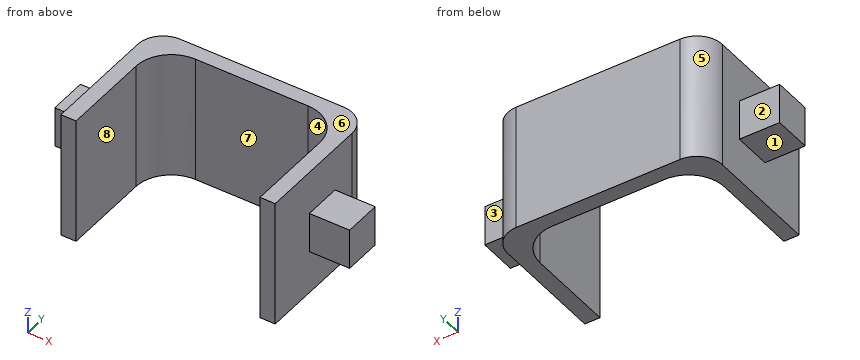
from build123d import *

# Parameters (mm, degrees)
BOSS_EXTRUDE1_DEPTH = 1.5875
BOSS_EXTRUDE2_DEPTH = 5
FILLET1_R           = 2
FILLET2_R           = 2
CUT_EXTRUDE1_DEPTH  = 10


with BuildPart() as part:
    # Sketch1 → Boss-Extrude1 (new body, symmetric)
    with BuildSketch(Plane.XY):
        Polygon((8.45, 11), (8.45, 7), (11.625, 7), (11.625, 4), (8.45, 4), (8.45, 0), (6.45, 0), (6.45, 9), (-6.45, 9), (-6.45, 0), (-8.45, 0), (-8.45, 4), (-11.625, 4), (-11.625, 7), (-8.45, 7), (-8.45, 11), align=None)
    extrude(amount=BOSS_EXTRUDE1_DEPTH, both=True)

    # Sketch2 → Boss-Extrude2 (add, symmetric)
    with BuildSketch(Plane.XY):
        Polygon((-8.45, 7), (-8.45, 4), (-8.45, 0), (-6.45, 0), (-6.45, 9), (6.45, 9), (6.45, 0), (8.45, 0), (8.45, 4), (8.45, 7), (8.45, 11), (-8.45, 11), align=None)
    extrude(amount=BOSS_EXTRUDE2_DEPTH, both=True)

    # Fillet1
    fillet1_edges = [part.edges().sort_by_distance(p)[0] for p in [
        (6.45, 9, 0),
        (-6.45, 9, 0),
    ]]
    fillet(fillet1_edges, radius=FILLET1_R)

    # Fillet2
    fillet2_edges = [part.edges().sort_by_distance(p)[0] for p in [
        (8.45, 11, 0),
        (-8.45, 11, 0),
    ]]
    fillet(fillet2_edges, radius=FILLET2_R)

    # Sketch3 → Cut-Extrude1 (cut)
    with BuildSketch(Plane.XY.offset(5)):
        with BuildLine():
            Line((7.25, 7), (7.25, 0))
            Line((7.25, 0), (6.45, 0))
            Line((6.45, 0), (6.45, 7))
            ThreePointArc((6.45, 7), (5.864213562, 8.414213562), (4.45, 9))
            Line((4.45, 9), (-4.45, 9))
            ThreePointArc((-4.45, 9), (-5.864213562, 8.414213562), (-6.45, 7))
            Line((-6.45, 7), (-6.45, 0))
            Line((-6.45, 0), (-7.25, 0))
            Line((-7.25, 0), (-7.25, 7))
            ThreePointArc((-7.25, 7), (-6.429898987, 8.979898987), (-4.45, 9.8))
            Line((-4.45, 9.8), (4.45, 9.8))
            ThreePointArc((4.45, 9.8), (6.429898987, 8.979898987), (7.25, 7))
        make_face()
    extrude(amount=-CUT_EXTRUDE1_DEPTH, mode=Mode.SUBTRACT)


solid = part.part
Input: part model. Units: mm. Frame: model coordinates. Face numbers are marked on the shaded views. A direction names the side the tool comes from. Round coordinates to 2 decimals unless told otherwise and drop trailing zeros. Write each loop counter-clockwise with the first axis right and the second up, starting at its lowest first coordinate (ties: lowest second). Pieces come first, ordered by that corner, then holes.
1) Ray query, L1, parallel to X at y = 2, z = 3.25; L2, parallel to Y at x = -3.25, z = 4.25; L3, parallel to X at y = 8.25, z = -2.25. Return the intervals inside material, ascending.
2) Cut plane D-D (x = 9.5). Return the cut outline in (y, z).
3) Draft query along X for the marked faces 5, 6, 7 and 8. Return one class per face: pulls with the +X half, pulls with the -X half, needs draft (parallel to the pull), parting line crosses it, or undercut.
4) Contact query for flat-ended pins moving along their axis: P1, Ø5, axis at y = 1, z = -3, coming from the +X side; P2, Ø1, axis at x = -0.5, z = 1, coming from the -Y side; P3, Ø1, axis at x = 10, z = 0, coming from the +Y side; P4, Ø5, axis at x = 3.5, y = 1.5, coming from the +Z side. Output: stop coordinate, or through.
5) Cut plane C-C (y = 1). Return the cut outline in (x, z).
6) Cut plane B-B (z = 0). Return the cut outline in (x, y) (3 decimals).
7) Reachability of the marked faces 1, 2, 3 and 4 from +Z, -Z, +X, -X, +Y, -Y: full face, straight path, thin tool, end or side. Return the list, or none.
Geometry says:
1. L1: x = -8.45 to -7.25, 7.25 to 8.45
1. L2: y = 9.8 to 11
1. L3: x = -8.45 to -6.96, 6.96 to 8.45
2. outline: (4, -1.59) - (7, -1.59) - (7, 1.59) - (4, 1.59) - close
3. face 5: pulls with the -X half
3. face 6: needs draft
3. face 7: undercut
3. face 8: undercut
4. P1: stops at x = 8.45
4. P2: stops at y = 9.8
4. P3: stops at y = 7
4. P4: passes through
5. outline: (-8.45, -5) - (-7.25, -5) - (-7.25, 5) - (-8.45, 5) - close; (7.25, -5) - (8.45, -5) - (8.45, 5) - (7.25, 5) - close
6. outline: (-11.625, 4) - (-8.45, 4) - (-8.45, 0) - (-7.25, 0) - (-7.25, 7) arc R2.8 cw to (-4.45, 9.8) - (4.45, 9.8) arc R2.8 cw to (7.25, 7) - (7.25, 0) - (8.45, 0) - (8.45, 4) - (11.625, 4) - (11.625, 7) - (8.45, 7) - (8.45, 9) arc R2 ccw to (6.45, 11) - (-6.45, 11) arc R2 ccw to (-8.45, 9) - (-8.45, 7) - (-11.625, 7) - close
7. face 1: -Z, -X, +Y, -Y
7. face 2: +Z, -Z, -X, +Y
7. face 3: +Z, -Z, +X, +Y
7. face 4: +Z, -Z, -Y
